```python
from build123d import *

# Parameters (mm, degrees)
RESSALTO_EXTRUS_O2_DEPTH = 50
CORTE_EXTRUS_O1_DEPTH    = 38
CORTE_EXTRUS_O3_DEPTH    = 47
ESBO_O5_W                = 1
ESBO_O5_H                = 8
CORTE_EXTRUS_O4_DEPTH    = 61.725636267
CORTE_EXTRUS_O5_DEPTH    = 7
CORTE_EXTRUS_O6_DEPTH    = 47


with BuildPart() as part:
    # Esboço1 → Ressalto-extrusão2 (new body)
    with BuildSketch(Plane(origin=(0, 0, 0), x_dir=(1, 0, 0), z_dir=(0, 1, 0))):
        with BuildLine():
            Line((-13.376104721, 16.054091922), (-22.876104721, -1.295908078))
            ThreePointArc((-22.876104721, -1.295908078), (-22.619735169, -16.393998269), (-9.5, -23.87))
            Line((-9.5, -23.87), (9.5, -23.87))
            ThreePointArc((9.5, -23.87), (22.619735169, -16.393998269), (22.876104721, -1.295908078))
            Line((22.876104721, -1.295908078), (13.376104721, 16.054091922))
            ThreePointArc((13.376104721, 16.054091922), (0, 23.98), (-13.376104721, 16.054091922))
        make_face()
    extrude(amount=RESSALTO_EXTRUS_O2_DEPTH)

    # Esboço3 → Corte-extrusão1 (cut)
    with BuildSketch(Plane.XZ):
        with BuildLine():
            Line((-9.5, 19.37), (9.5, 19.37))
            ThreePointArc((9.5, 19.37), (18.748337906, 14.100031567), (18.929057426, 3.45711553))
            Line((18.929057426, 3.45711553), (9.429057426, -13.89288447))
            ThreePointArc((9.429057426, -13.89288447), (0, -19.48), (-9.429057426, -13.89288447))
            Line((-9.429057426, -13.89288447), (-18.929057426, 3.45711553))
            ThreePointArc((-18.929057426, 3.45711553), (-18.748337906, 14.100031567), (-9.5, 19.37))
        make_face()
    extrude(amount=-CORTE_EXTRUS_O1_DEPTH, mode=Mode.SUBTRACT)

    # Esboço4 → Corte-extrusão3 (cut)
    with BuildSketch(Plane.XZ):
        with BuildLine():
            Line((0, 3.37), (18.88135728, 3.37))
            Line((18.88135728, 3.37), (9.429057426, -13.89288447))
            ThreePointArc((9.429057426, -13.89288447), (0, -19.48), (-9.429057426, -13.89288447))
            Line((-9.429057426, -13.89288447), (-18.88135728, 3.37))
            Line((-18.88135728, 3.37), (0, 3.37))
        make_face()
    extrude(amount=-CORTE_EXTRUS_O3_DEPTH, mode=Mode.SUBTRACT)

    # Esboço5 → Corte-extrusão4 (cut, through all)
    with BuildSketch(Plane(origin=(0, 0, 0), x_dir=(-1, 0, 0), z_dir=(0, -1, 0))):
        with Locations((-5.5, 7.13)):
            Rectangle(ESBO_O5_W, ESBO_O5_H)
        with Locations((5.5, 7.13)):
            Rectangle(ESBO_O5_W, ESBO_O5_H)
    extrude(amount=-CORTE_EXTRUS_O4_DEPTH, mode=Mode.SUBTRACT)

    # Esboço6 → Corte-extrusão5 (cut)
    with BuildSketch(Plane.XZ):
        Polygon((-13.774214885, -10.63), (13.780859913, -10.63), (19.256364236, -0.63), (2.792834358, -0.63), (-19.234396653, -0.63), align=None)
    extrude(amount=-CORTE_EXTRUS_O5_DEPTH, mode=Mode.SUBTRACT)

    # Esboço7 → Corte-extrusão6 (cut)
    with BuildSketch(Plane.XZ):
        Polygon((0, -12.48), (13, -12.48), (13, -8.48), (-13, -8.48), (-13, -12.48), align=None)
    extrude(amount=-CORTE_EXTRUS_O6_DEPTH, mode=Mode.SUBTRACT)


solid = part.part
```
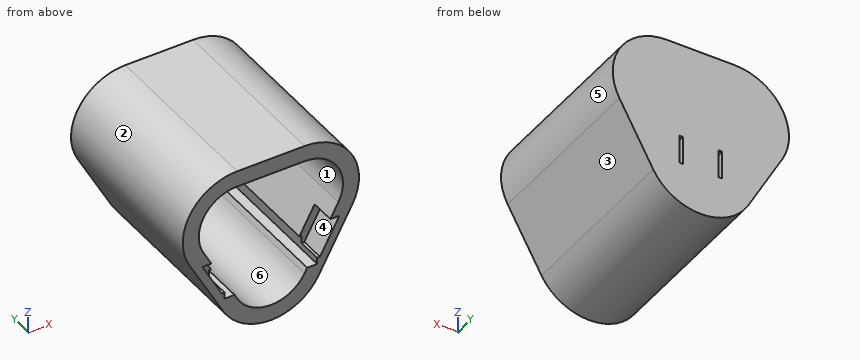
Source: CAD feature listing. Evaluate the final solid. Frame: model axes, mm. Face numbers are marked on the shaded views. A direction names the side the tool comes from. Coordinates: 2 decimals unless noted, no trailing zeros. Loops run counter-clockwise (first coordinate to the right, second up) from the corner with the lowest first, then second, coordinate; pieces in that order, holes last. Notation, with made-up numbers: M 0,34 L 47,34 A22 cw 47,48 Z; hole C 21,47.5 d6. An arc over 180 degrees is marked long. Use a Markdown table: item, result. Add a question column.
Q1. Section query B-B, the plane z = 5. Return loops of the section in (x, y), and give its area (3 significant figures).
Q2. Material intervals for L1, parallel to Z at x = 0, y = 36.5; L2, parallel to Z at x = 12.5, y = 24; L3, parallel to Z at x = 17.5, y = 4, sorted ascending.
Q3. Section query C-C, the plane x = 4. Return loops of the section in (y, z), and give its area (3 significant figures).
Q4. Draft query along X for the marked faces 1, 2, 3 and 4. Return one class per face: pulls with the +X half, pulls with the -X half, needs draft (parallel to the pull), parting line crosses it, or undercut.
Q5. Access query for the marked faces 5 and 6. Directions: +Z, -Z, +X, -X, +Y, -Y. A direction counts if a zero-diameter tool reaches every point of the face in a straight line with its end or side. Return the directions, or none.
Q6. First-contact query: pin 1 (1.2 mm diameter, centred on y = 24, z = -10.5, fed in from -X); pin 2 (10 mm diameter, centred on y = 5.5, z = 14, fed in from +X); pin 3 (2 mm diameter, centred on x = 18.5, y = 3, fed in from -Z). Flat tips, straight axial feed; report the tip coordinate or a pass-through.
Q7. Section query A-A, the plane y = 41. Return loops of the section in (x, z).
Q8. Section query D-D, the plane y = 36. Return loops of the section in (x, z).
Result:
| question | item | result |
|---|---|---|
| 1 | outline | M -24.31,0 L -19.62,0 L -19.62,38 L 19.62,38 L 19.62,0 L 24.31,0 L 24.31,50 L -24.31,50 Z |
| 1 | area | 940 mm2 |
| 2 | L1 | z = -23.98 to -19.48, 19.37 to 23.87 |
| 2 | L2 | z = -17.47 to -12.48, -8.48 to -8.28, 18.94 to 23.57 |
| 2 | L3 | z = -8.52 to -3.84, -0.63 to 0.85, 15.8 to 21.6 |
| 3 | outline | M 0,-23.45 L 50,-23.45 L 50,23.87 L 0,23.87 L 0,19.37 L 38,19.37 L 38,3.37 L 47,3.37 L 47,-18.71 L 0,-18.71 Z |
| 3 | area | 720 mm2 |
| 4 | face 1 | undercut |
| 4 | face 2 | pulls with the -X half |
| 4 | face 3 | pulls with the +X half |
| 4 | face 4 | undercut |
| 5 | face 5 | +X, +Y, -Y |
| 5 | face 6 | -Y |
| 6 | pin 1 | stops at x = -16.75 |
| 6 | pin 2 | stops at x = 24.75 |
| 6 | pin 3 | stops at z = -8.52 |
| 7 | outline | M -22.88,1.3 L -13.38,-16.05 A15.25 ccw 13.38,-16.05 L 22.88,1.3 A15.25 ccw 9.5,23.87 L -9.5,23.87 A15.25 ccw Z; hole M -18.88,3.37 L -12.39,-8.48 L -13,-8.48 L -13,-12.48 L -10.2,-12.48 L -9.43,-13.89 A10.75 ccw 9.43,-13.89 L 10.2,-12.48 L 13,-12.48 L 13,-8.48 L 12.39,-8.48 L 18.88,3.37 Z |
| 8 | outline | M -22.88,1.3 L -13.38,-16.05 A15.25 ccw 13.38,-16.05 L 22.88,1.3 A15.25 ccw 9.5,23.87 L -9.5,23.87 A15.25 ccw Z; hole M -18.93,3.46 L -12.39,-8.48 L -13,-8.48 L -13,-12.48 L -10.2,-12.48 L -9.43,-13.89 A10.75 ccw 9.43,-13.89 L 10.2,-12.48 L 13,-12.48 L 13,-8.48 L 12.39,-8.48 L 18.93,3.46 A10.75 ccw 9.5,19.37 L -9.5,19.37 A10.75 ccw Z |
